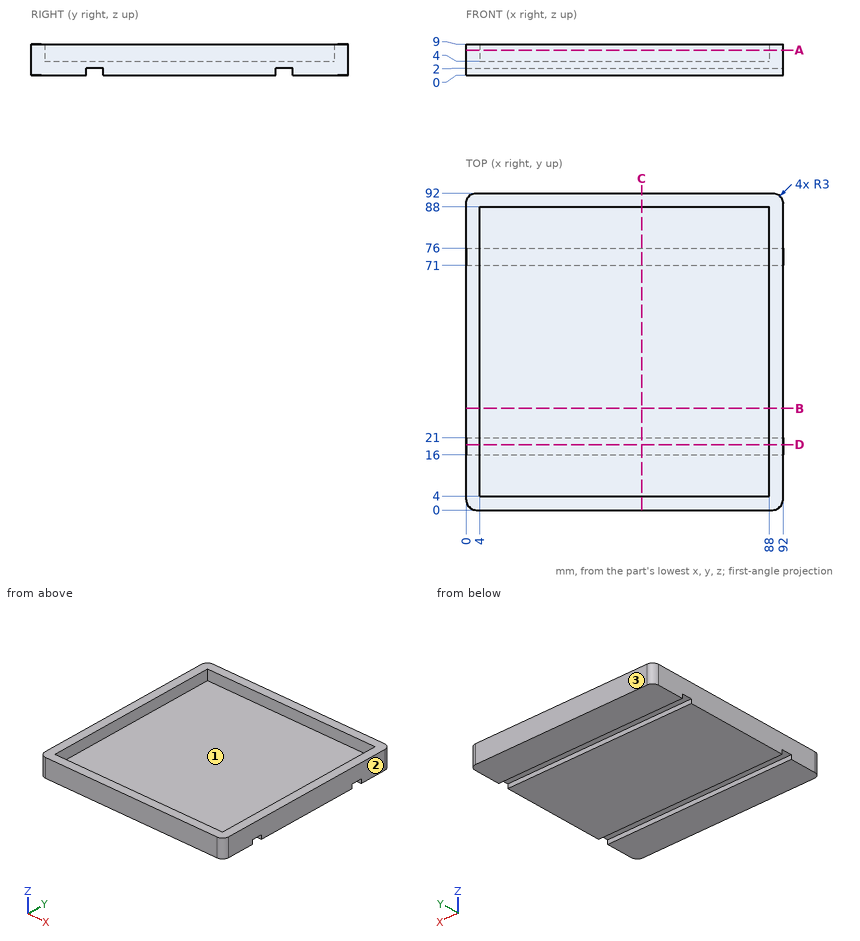
Study the drawing (mm; zero at the part's minimum x, y, z) and answer. Coordinates: 2 decimals unless noted, no trailing zeros. Write each loop counter-clockwise with the first axis right and the second up, starting at its lowest first coordinate (ties: lowest second). Pieces come first, ordered by that corner, then holes. Notation, with made-up numbers: (-16, 27) - (22, 27) arc R33 cw to (22, 58) - close; hole circle Ø1 at (-37, -38). An arc over 180 degrees is marked (long way). Answer as a JSON object with one key per item and string values. Group by question number.
1. A cutting plane is placed at A-A (z = 7.25). Determine the outline of the cut face in (x, y), plus the area to 3 significant figures.
2. Consider L1, parallel to Y at x = 66, z = 0.75; L2, parallel to Y at x = 49, z = 7.25. Determine where each line is inside the solid, lowest interval first. Write a range as [from, to].
3. The mould has two halves that part along Y. Classify the marked faces 1, 2 and 3: +Y half, -Y half, draft (parallel to the pull), parting line (faces both ways), or undercut.
4. A cutting plane is placed at B-B (y = 29.5). Determine the outline of the cut face in (x, z), plus the area to 3 significant figures.
5. A cutting plane is placed at C-C (x = 51). Determine the outline of the cut face in (y, z).
6. A cutting plane is placed at D-D (y = 19). Determine the outline of the cut face in (x, z), plus the area to 3 significant figures.
7. Each of these flat-tipped pins is pushed along its axis until it touches: P1, Ø10, axis at x = 46.5, y = 78, coming from the +Z side; P2, Ø2.5, axis at x = 59, y = 18.5, coming from the -Z side. Where does it stop, or does it pass through?
Worked out:
{
 "1": {"outline": "(0, 3) arc R3 ccw to (3, 0) - (89, 0) arc R3 ccw to (92, 3) - (92, 89) arc R3 ccw to (89, 92) - (3, 92) arc R3 ccw to (0, 89) - close; hole (4, 4) - (88, 4) - (88, 88) - (4, 88) - close", "area": "1,400 mm²"},
 "2": {"L1": "y = [0, 16], [21, 71], [76, 92]", "L2": "y = [0, 4], [88, 92]"},
 "3": {"face 1": "undercut", "face 2": "draft", "face 3": "+Y half"},
 "4": {"outline": "(0, 0) - (92, 0) - (92, 9) - (88, 9) - (88, 4) - (4, 4) - (4, 9) - (0, 9) - close", "area": "408 mm²"},
 "5": {"outline": "(0, 0) - (16, 0) - (16, 2) - (21, 2) - (21, 0) - (71, 0) - (71, 2) - (76, 2) - (76, 0) - (92, 0) - (92, 9) - (88, 9) - (88, 4) - (4, 4) - (4, 9) - (0, 9) - close"},
 "6": {"outline": "(0, 2) - (92, 2) - (92, 9) - (88, 9) - (88, 4) - (4, 4) - (4, 9) - (0, 9) - close", "area": "224 mm²"},
 "7": {"P1": "stops at z = 4", "P2": "stops at z = 2"}
}
